Build history of the part. All positions in model axes, mm. A direction names the side the tool comes from. Coordinates: 2 decimals unless noted, no trailing zeros. Loops run counter-clockwise (first coordinate to the right, second up) from the corner with the lowest first, then second, coordinate; pieces in that order, holes last.
(1) Slice it at D-D (y = -7.25). Give the cut face in (x, z), and give its area (3 significant figures).
(2) Wall check: L1, parallel to Y at x = 1.25, z = 1.45; L2, parallel to Z at x = 0.1, y = -1.25. Give the ranges that are in metal, low to high.
(3) Flat gauge pins, fed straight in: P1, Ø1.5, axis at x = -1, y = -5.5, coming from the +Z side; P2, Ø1, axis at x = -0.5, z = 1, coming from the -Y side; P3, Ø2, axis at x = 1, z = 1, coming from the -Y side. Where does each tip first touch, or does it go through?
(4) Slice it at B-B (x = 0). Give the cut face in (y, z).
(5) Slice it at C-C (y = 2.5). Give the cut face in (x, z).
(6) Two-plate mould, pull along Y, no slides. Class faces 3 (the face through (-1, -1, -1)), 4 (the face through (-0.91, -8.27, 0.7)), 5 (the face through (0, 5, 0)): pulls with the +Y half, pulls with the -Y half, needs draft (parallel to the pull), parting line crosses it, or undercut.
(7) Slice it at A-A (z = 0). Give the cut face in (x, y), and give its area (3 significant figures).
(8) Tool access for faces 1 (the face through (-0.63, 2.47, -0.49)), 2 (the face through (0.434, -0.493, -1.952)): list every direction of +Z, -Z, +X, -X, +Y, -Y with a clear straight run to the whole face (end or side of a thin tool).
Autodesk Inventor part; units mm, degrees
ref_plane "YZ Plane" through (0, 0, 0) normal (1, 0, 0) x (0, 1, 0)
ref_plane "XZ Plane" through (0, 0, 0) normal (0, 1, 0) x (-1, 0, 0)
ref_plane "XY Plane" through (0, 0, 0) normal (0, 0, 1) x (1, 0, 0)
sketch "Sketch1" plane through (0, 0, 0) normal (0, 1, 0) x (-1, 0, 0)
  circle A0 centre (0, 0) radius 2
  dimension "d0" = 4
extrude "Extrusion1" add sketch "Sketch1" against normal blind 1
sketch "Sketch2" plane through (0, 0, 0) normal (0, 1, 0) x (1, 0, 0)
  circle A0 centre (0, 0) radius 0.8
  dimension "d4" = 1.6
extrude "Extrusion2" add sketch "Sketch2" along normal blind 5
thread "Thread1"
sketch "Sketch3" plane through (0, -1, 0) normal (0, -1, 0) x (1, 0, 0)
  circle A0 centre (0, 0) radius 1.15
  dimension "d9" = 2.3
extrude "Extrusion3" add sketch "Sketch3" along normal blind 15.9
fillet "Fillet2" radius 1.15 1 edges at (-1.15, -16.9, 0)
sketch "Sketch4" plane through (0, 0, 0) normal (0, 0, 1) x (1, 0, 0)
  line L0 (-2, -1) -> (2, -1)
  line L1 (2, 0) -> (-2, 0)
  line L2 (0.8, 5) -> (-0.8, 5)
  line L3 (-0.8, 0) -> (0.8, 0)
  line L4 (0.8, 0) -> (0.6, 0)
  line L5 (0.6, 0) -> (0.6, 0.2)
  line L6 (0.6, 0.2) -> (0.8, 0.2)
  line L7 (0.8, 0.2) -> (0.8, 0)
  line L8 (0, -2.2) -> (0, 6.2)
  point P0 (0, 0)
  dimension "d13" = 0.2
  dimension "d14" = 0.2
revolve "Revolution1" cut sketch "Sketch4" angle 360 about axis through (0, -10, 0) along (0, 1, 0)
chamfer "Chamfer1" distance 0.2 angle 45 1 edges at (-0.8, 5, 0)
equation "\"d12\" = 0.5 * d9"
properties part number "KN-00-03-01" material "X105CrMo17"
Response values:
1. outline: circle Ø2.3 at (0, 0)
1. area: 4.15 mm2
2. L1: y = -1 to 0
2. L2: z = -1.15 to 1.15
3. P1: stops at z = 1.12
3. P2: stops at y = -16.72
3. P3: stops at y = -16.82
4. outline: (-15.75, -1.15) - (-1, -1.15) - (-1, -2) - (0, -2) - (0, -0.6) - (0.2, -0.6) - (0.2, -0.8) - (4.8, -0.8) - (5, -0.6) - (5, 0.6) - (4.8, 0.8) - (0.2, 0.8) - (0.2, 0.6) - (0, 0.6) - (0, 2) - (-1, 2) - (-1, 1.15) - (-15.75, 1.15) arc R1.15 ccw to start
5. outline: circle Ø1.6 at (0, 0)
6. face 3: pulls with the -Y half
6. face 4: needs draft
6. face 5: pulls with the +Y half
7. outline: (-2, -1) - (-1.15, -1) - (-1.15, -15.75) arc R1.15 ccw to (1.15, -15.75) - (1.15, -1) - (2, -1) - (2, 0) - (0.6, 0) - (0.6, 0.2) - (0.8, 0.2) - (0.8, 4.8) - (0.6, 5) - (-0.6, 5) - (-0.8, 4.8) - (-0.8, 0.2) - (-0.6, 0.2) - (-0.6, 0) - (-2, 0) - close
7. area: 47.9 mm2
8. face 1: +Y
8. face 2: +Y, -Y
